from build123d import *

# Parameters (mm, degrees)
F1_DEPTH  = 28.575
F2_R      = 2.38125
F3_DEPTH  = 12.7
F4_W      = 21.6915998608
F4_H      = 22.372465115
F4_H_2    = 22.0895758063
F5_DEPTH  = 11.176
F6_R      = 2.38125
F7_DEPTH  = 21.6915998608
F8_W      = 17.9831998608
F8_H      = 49.9544155288
F9_DEPTH  = 23.5458
F11_DEPTH = 9.2202


with BuildPart() as f1:
    # F0 (on Front) → F1 (new body, symmetric)
    with BuildSketch(Plane.XZ):
        Polygon((-12.7, 25.4), (-12.7, 0), (12.7, 0), (12.7, 25.4), (10.8457999304, 25.4), (10.8457999304, 1.8542000696), (-10.8457999304, 1.8542000696), (-10.8457999304, 25.4), align=None)
    extrude(amount=F1_DEPTH, both=True)

    # F2 (on Right) → F3 (cut, symmetric)
    with BuildSketch(Plane.YZ):
        with BuildLine():
            ThreePointArc((15.875, 25.4), (24.8552561211, 21.6802561211), (28.575, 12.7))
            Line((28.575, 12.7), (28.575, 25.4))
            Line((28.575, 25.4), (15.875, 25.4))
        make_face()
        with BuildLine():
            ThreePointArc((28.575, 12.7), (24.8552561211, 3.7197438789), (15.875, 0))
            Line((15.875, 0), (28.575, 0))
            Line((28.575, 0), (28.575, 12.7))
        make_face()
        with BuildLine():
            ThreePointArc((-15.875, 0), (-24.8552561211, 3.7197438789), (-28.575, 12.7))
            Line((-28.575, 12.7), (-28.575, 0))
            Line((-28.575, 0), (-15.875, 0))
        make_face()
        with BuildLine():
            ThreePointArc((-28.575, 12.7), (-24.8552561211, 21.6802561211), (-15.875, 25.4))
            Line((-15.875, 25.4), (-28.575, 25.4))
            Line((-28.575, 25.4), (-28.575, 12.7))
        make_face()
        with Locations((-15.875, 12.7)):
            Circle(F2_R)
        with Locations((15.875, 12.7)):
            Circle(F2_R)
    extrude(amount=F3_DEPTH, both=True, mode=Mode.SUBTRACT)

    # F4 (on face) → F5 (cut)
    with BuildSketch(Plane.XY.offset(1.8542000696)):
        with Locations((0, 17.5362325575)):
            Rectangle(F4_W, F4_H)
        with Locations((0, -17.3947879031)):
            Rectangle(F4_W, F4_H_2)
    extrude(amount=-F5_DEPTH, mode=Mode.SUBTRACT)

    # F6 (on face) → F7 (join, through all)
    with BuildSketch(Plane.YZ.offset(-10.8457999304)):
        with BuildLine():
            Line((-12.7, 25.4), (-43.815, 25.4))
            ThreePointArc((-43.815, 25.4), (-52.7952561211, 21.6802561211), (-56.515, 12.7))
            ThreePointArc((-56.515, 12.7), (-52.7952561211, 3.7197438789), (-43.815, 0))
            Line((-43.815, 0), (-12.7, 0))
            ThreePointArc((-12.7, 0), (-3.7197438789, 3.7197438789), (0, 12.7))
            ThreePointArc((0, 12.7), (-3.7197438789, 21.6802561211), (-12.7, 25.4))
        make_face()
        with Locations((-43.815, 12.7)):
            Circle(F6_R, mode=Mode.SUBTRACT)
        with Locations((-15.875, 12.7)):
            Circle(F6_R, mode=Mode.SUBTRACT)
    extrude(amount=F7_DEPTH)

    # F8 (on face) → F9 (cut)
    with BuildSketch(Plane(origin=(0, 0, 0), x_dir=(1, 0, 0), z_dir=(0, 0, -1))):
        with Locations((0, 31.4859015796)):
            Rectangle(F8_W, F8_H)
    extrude(amount=-F9_DEPTH, mode=Mode.SUBTRACT)

    # F10 (on Right) → F11 (cut, symmetric)
    with BuildSketch(Plane.YZ):
        with BuildLine():
            Line((-31.75, 25.4), (-43.815, 25.4))
            ThreePointArc((-43.815, 25.4), (-56.515, 12.7), (-43.815, 0))
            Line((-43.815, 0), (-12.7, 0))
            ThreePointArc((-12.7, 0), (0, 12.7), (-12.7, 25.4))
            Line((-12.7, 25.4), (-19.05, 25.4))
            Line((-19.05, 25.4), (-19.05, 23.5204))
            Line((-19.05, 23.5204), (-31.75, 23.5204))
            Line((-31.75, 23.5204), (-31.75, 25.4))
        make_face()
    extrude(amount=F11_DEPTH, both=True, mode=Mode.SUBTRACT)


solid = f1.part
Model file for the job. Use its own axes, mm. A direction names the side the tool comes from. Give positions to 0.01 mm unless a question says otherwise; leave off trailing zeros. Order: outer loops, then holes, each group sorted by start corner. A loop starts at its lowest first (then second) coordinate and runs counter-clockwise, first axis right, second up. Notation, with made-up numbers: M -4,85 L 3,85 A27 cw 3,108 Z; hole C 43,59.5 d10. An arc over 180 degrees is marked long. Write item = value, one per line.
Q1. Cut at A-A, the plane x = 4. List the corners of the cut face in (y, z), then the cut area to 3 significant figures.
Derived:
outline = M -31.75,23.55 L -19.05,23.55 L -19.05,25.4 L -31.75,25.4 Z; M -6.35,0 L 6.35,0 L 6.35,1.85 L -6.09,1.85 A12.7 cw -6.35,1.7 Z
area = 47.1 mm2
Q2. Cut at D-D, the plane z = 20.5. List the corners of the cut face in (x, y).
Derived:
outline = M -12.7,-25.9 L -10.85,-25.9 L -10.85,-53.84 L -9.22,-53.84 L -9.22,-2.68 L -10.85,-2.68 L -10.85,25.9 L -12.7,25.9 Z; M 9.22,-53.84 L 10.85,-53.84 L 10.85,-25.9 L 12.7,-25.9 L 12.7,25.9 L 10.85,25.9 L 10.85,-2.68 L 9.22,-2.68 Z
Q3. Flat gauge pins, fed straight in: pin 1 (1.5 mm diameter, centred on x = -3, z = 24, fed in from +Y); pin 2 (12 mm diameter, centred on y = -35.5, z = 19.5, fed in from -X); pin 3 (1.5 mm diameter, centred on x = -4, z = 25, fed in from -Y). Where does each tip first touch, or does it go through?
Derived:
pin_1 = -19.05
pin_2 = -10.85
pin_3 = -31.75
Q4. Drill centre lines: line 1 (Y direction, x = 10.4, z = 12.7) (3 decimals); line 2 (X direction, y = 18.5, z = 6.25); line 3 (X direction, y = -26, z = 1.5). Where is each one in solid material? Low to high. Write a range as [from, to].
Derived:
line_1 = [-56.515, -46.196], [-41.434, -18.256], [-13.494, 0]
line_2 = [-12.7, -10.85], [10.85, 12.7]
line_3 = [-10.85, -9.22], [9.22, 10.85]
Q5. Cut at B-B, the plane y = -34.5. List the corners of the cut face in (x, z).
Derived:
outline = M -10.85,0 L -9.22,0 L -9.22,25.4 L -10.85,25.4 Z; M 9.22,0 L 10.85,0 L 10.85,25.4 L 9.22,25.4 Z
Q6. Tool access for faces 1 (the flat face through (0, -31.75, 24)), 2 (the cylindrical face through (-11.76, 18.146, 13.415)), 3 (the flat face through (-10.846, -7.9, 0.5)): list every direction of +Z, -Z, +X, -X, +Y, -Y with a clear straight run to the whole face (end or side of a thin tool).
Derived:
face_1 = +Z, -Z, -Y
face_2 = +X, -X
face_3 = -Z
Q7. Cut at C-C, the plane y = 8.5. List the corners of the cut face in (x, z).
Derived:
outline = M -12.7,0 L -10.85,0 L -10.85,25.4 L -12.7,25.4 Z; M 10.85,0 L 12.7,0 L 12.7,25.4 L 10.85,25.4 Z
Q8. Two-plate mould, pull along Y, no slides. Class faces 4 (the flat face through (0, -25, 23.546)), 5 (the cylindrical face through (-10.044, -46.194, 12.805)), 6 (the flat face through (0, 6.35, 1)): pulls with the +Y half, pulls with the -Y half, needs draft (parallel to the pull), parting line crosses it, or undercut.
Derived:
face_4 = needs draft
face_5 = undercut
face_6 = pulls with the +Y half
